Autodesk Inventor part; units mm, degrees
ref_plane "YZ Plane" through (0, 0, 0) normal (1, 0, 0) x (0, 1, 0)
ref_plane "XZ Plane" through (0, 0, 0) normal (0, 1, 0) x (-1, 0, 0)
ref_plane "XY Plane" through (0, 0, 0) normal (0, 0, 1) x (1, 0, 0)
sketch "Szkic1" plane through (0, 0, 0) normal (0, 1, 0) x (-1, 0, 0)
  circle A0 centre (0, 0) radius 14.1 construction
  line L0 (0, 0) -> (-14.1, 0) construction
  circle A1 centre (0, 0) radius 22.5 construction
  circle A2 centre (-13.2497, 4.8225) radius 1.75
  circle A3 centre (-13.2497, -4.8225) radius 1.75
  circle A4 centre (2.4484, 13.8858) radius 1.75
  circle A5 centre (10.8012, 9.0633) radius 1.75
  circle A6 centre (10.8012, -9.0633) radius 1.75
  circle A7 centre (2.4484, -13.8858) radius 1.75
  circle A8 centre (0, 0) radius 35
  circle A9 centre (-13.2497, 4.8225) radius 3.25
  circle A10 centre (-13.2497, -4.8225) radius 3.25
  circle A11 centre (2.4484, -13.8858) radius 3.25
  circle A12 centre (10.8012, -9.0633) radius 3.25
  circle A13 centre (10.8012, 9.0633) radius 3.25
  circle A14 centre (2.4484, 13.8858) radius 3.25
  line L1 (12.4262, 11.8779) -> (4.0734, 16.7004)
  line L2 (9.1762, 6.2487) -> (0.8234, 11.0712)
  line L3 (-9.9997, 4.8225) -> (-9.9997, -4.8225)
  line L4 (12.4262, -11.8779) -> (4.0734, -16.7004)
  line L5 (9.1762, -6.2487) -> (0.8234, -11.0712)
  line L6 (-16.4997, -4.8225) -> (-16.4997, 4.8225)
  line L7 (-40, 35) -> (40, 35)
  line L8 (40, 35) -> (40, -35)
  line L9 (40, -35) -> (-40, -35)
  line L10 (-40, -35) -> (-40, 35)
  line L11 (-40, 35) -> (40, -35) construction
  line L12 (40, 35) -> (-40, -35) construction
  line L13 (0, -35) -> (0, 35)
  line L14 (40, 0) -> (-40, 0)
  line L15 (56, 0) -> (-56, 0)
  point P0 (0, -35)
  point P1 (0, 35)
  point P2 (35, 0)
  point P3 (-35, 0)
  dimension "d0" = 28.2
  dimension "d1" = 3.5
  dimension "d2" = 40
  dimension "d5" = 360
  dimension "d7" = 45
  dimension "d8" = 70
  dimension "d12" = 6.5
  dimension "d15" = 360
  dimension "d27" = 80
  dimension "d28" = 70
revolve "Obrót2" add sketch "Szkic1" angle 180 about axis through (-10, 0, 0) along (-1, 0, 0) contours A2 | A4 | A5 | L14 L13 A14 L2 A13 L1 A8 | A8 L7 L8 L14 | L13 A14 L14 L3 A9 L6 A8 | A8 L14 L10 L7 | L13 A14 | A14 L13 | L14 L6 A9 L3 | L1 A13 L2 A14 | A9 | A13
extrude "Wyciągnięcie proste1" cut sketch "Szkic1" along normal through all contours A2 | A3 | A4 | A5 | A6 | A7 | L13 A14 | A14 L13 | L13 A11 | A11 L13 | L14 L6 A9 L3 | L3 A10 L6 L14 | L1 A13 L2 A14 | A11 L5 A12 L4 | A9 | A10 | A13 | A12
extrude "Wyciągnięcie proste2" add sketch "Szkic1" along normal blind 17.85 contours L13 A14 | A14 L13 | L13 A11 | A11 L13 | L14 L6 A9 L3 | L3 A10 L6 L14 | L1 A13 L2 A14 | A11 L5 A12 L4 | A9 | A10 | A13 | A12
extrude "Wyciągnięcie proste3" cut sketch "Szkic1" along normal blind 7.85 contours A2 | A3 | A4 | A5 | A6 | A7 | L14 L13 A14 L2 A13 L1 A8 | L14 L8 L9 A8 | A8 L7 L8 L14 | A8 L13 A11 L4 A12 L5 L14 | L13 A14 L14 L3 A9 L6 A8 | A8 L14 L10 L7 | L9 L10 L14 A8 | A8 L14 L6 A10 L3 L13 A11 | L13 A14 | A14 L13 | L13 A11 | A11 L13 | L14 L6 A9 L3 | L3 A10 L6 L14 | L1 A13 L2 A14 | A11 L5 A12 L4 | A9 | A10 | A13 | A12
fillet "Zaokrąglenie1" radius 2 2 edges at (-40, 35, 0) (40, 35, 0)
properties part number "semicylinder_2"
Read the model definition and answer for the solid it produces. Units are mm, in the model's axes. A direction names the side the tool comes from. Round coordinates to 2 decimals unless told otherwise and drop trailing zeros. Order: outer loops, then holes, each group sorted by start corner. A loop starts at its lowest first (then second) coordinate and runs counter-clockwise, first axis right, second up.
1) The mould has two halves that part along X. Classify faces 1 (the face through (40, 18, 0)), 2 (the face through (-8.308, 25.281, 14.255)), 3 (the face through (-40, 18, 0)): released by +X, released by -X, zero draft, split by the parting line, or undercut.
2) For faces 4 (the face through (-10.422, 12.78, -7.355)), 5 (the face through (0.33, 25.42, -15.57)), determine the directions among +Z, -Z, +X, -X, +Y, -Y from which every point of the face is accessible in a straight line to the end or side of a thin tool.
3) The part is cut by section B-B on y = 11.5. Give the number of separate pieces and of enclosed holes in the cut face, plus the area to 3 significant figures.
4) Straight lines are drawn through the part: L1, parallel to X at y = 19.5, z = -7; L2, parallel to X at y = 11, z = 5; L3, parallel to Y at x = 24.5, z = -1. For each, find the intervals that lie inside material, in ascending order.
5) Flat-ended cylindrical pins translate along their axes: pin 1 (1.5 mm diameter, centred on x = 10.5, y = 17.5, fed in from -Z); pin 2 (5.5 mm diameter, centred on x = -6, z = -10.5, fed in from +Y); pin 3 (10 mm diameter, centred on x = 23, z = 12.5, fed in from +Y). Find the tip coordinate at first contact, or state that the pin passes through.
6) The part is cut by section A-A on x = 18. Write down the section's boundary in (y, z), plus the area to 3 significant figures.
Resolved:
1. face 1: released by +X
1. face 2: undercut
1. face 3: released by -X
2. face 4: +Y, -Y
2. face 5: +Y
3. separate pieces: 1
3. enclosed holes: 6
3. area: 5,230 mm2
4. L1: x = -40 to -13.31, -7.87 to 10.84, 15.66 to 40
4. L2: x = -40 to 11.51, 14.99 to 40
4. L3: y = 7.85 to 34.99
5. pin 1: stops at z = -30.73
5. pin 2: stops at y = 34.13
5. pin 3: stops at y = 34.19
6. outline: (7.85, -34.11) arc R35 ccw to (7.85, 34.11) - close
6. area: 1,380 mm2
